For this review, take the finished solid that the model builds, in its own axes (mm). Coordinates: 2 decimals unless noted, no trailing zeros. Loops run counter-clockwise (first coordinate to the right, second up) from the corner with the lowest first, then second, coordinate; pieces in that order, holes last.
```python
from build123d import *

# Parameters (mm, degrees)
F1_DEPTH     = 2
F3_DEPTH     = 40
F4_T1_DEPTH  = 40
F4_T3_DEPTH  = 90
F4_T5_DEPTH  = 20
F4_T8_ANGLE  = 90
F4_T10_ANGLE = 90
F4_T12_ANGLE = 90
F4_T14_ANGLE = 90
F4_T15_DEPTH = 20
F4_T17_DEPTH = 34.8706177507
F4_T19_DEPTH = 34.8706177507
F4_T22_ANGLE = 90
F4_T24_ANGLE = 90
F4_T26_ANGLE = 90
F4_T28_ANGLE = 90
F4_T32_ANGLE = 67.9058899257
F4_S33_R     = 4
F4_T34_DEPTH = 6
F4_T38_ANGLE = 67.9058899257
F4_S39_R     = 4
F4_T40_DEPTH = 6
F4_T42_ANGLE = 2.1985680139
F4_T44_ANGLE = 2.1985680139
F4_T46_ANGLE = 145.4380511244
F4_T48_ANGLE = 145.4380511244
F5_W         = 47.7962438017
F5_H         = 14.3843935803
F6_DEPTH     = 25
F7_W         = 52.0751457661
F7_H         = 31.3179213554
F8_DEPTH     = 25


# Not quite as in the source:
# - a fillet or chamfer that OpenCascade refuses, or shapes differently, is made with other operations: its cross-section is extruded or revolved along the edge and cut away or added


with BuildPart() as f1:
    # F0 (on Top) → F1 (new body)
    with BuildSketch(Plane.XY):
        with BuildLine():
            Line((45, 20), (-45, 20))
            ThreePointArc((-45, 20), (-52.0710678119, 17.0710678119), (-55, 10))
            Line((-55, 10), (-55, -10))
            ThreePointArc((-55, -10), (-52.0710678119, -17.0710678119), (-45, -20))
            Line((-45, -20), (45, -20))
            ThreePointArc((45, -20), (52.0710678119, -17.0710678119), (55, -10))
            Line((55, -10), (55, 10))
            ThreePointArc((55, 10), (52.0710678119, 17.0710678119), (45, 20))
        make_face()
    extrude(amount=F1_DEPTH)

    # F2 (on face) → F3 (join, through all)
    with BuildSketch(Plane(origin=(0, 20, 0), x_dir=(-1, 0, 0), z_dir=(0, 1, 0))):
        with BuildLine():
            ThreePointArc((2.7771054409, 7.1347622527), (0, 3), (-2.7771054409, 7.1347622527))
            ThreePointArc((-2.7771054409, 7.1347622527), (-3.0758368725, 7.6594328143), (-3.674432988, 7.5806777712))
            ThreePointArc((-3.674432988, 7.5806777712), (-3.9185059144, 6.8033127653), (-3.9999931862, 5.9926169097))
            ThreePointArc((-3.9999931862, 5.9926169097), (-6.509106512, 3.1485501635), (-10.1236877963, 2))
            Line((-10.1236877963, 2), (10.1236877963, 2))
            ThreePointArc((10.1236877963, 2), (6.509106512, 3.1485501635), (3.9999931862, 5.9926169097))
            ThreePointArc((3.9999931862, 5.9926169097), (3.9185059144, 6.8033127653), (3.674432988, 7.5806777712))
            ThreePointArc((3.674432988, 7.5806777712), (3.0758368725, 7.6594328143), (2.7771054409, 7.1347622527))
        make_face()
    extrude(amount=-F3_DEPTH)

    # F4: fillet of radius 0.3 on 22 edges, made by hand

    # F4_s2 → F4_t1 (join)
    with BuildSketch(Plane.XZ.offset(-20)):
        with BuildLine():
            ThreePointArc((10.1293822493, 2), (10.1236267648, 2.0000552144), (10.1178733989, 2.0002208373))
            ThreePointArc((10.1178733989, 2.0002208373), (10.120780575, 2.0001098236), (10.1236877963, 2))
            Line((10.1236877963, 2), (10.1293822493, 2))
        make_face()
        with BuildLine():
            ThreePointArc((-10.1293822493, 2), (-10.1236267648, 2.0000552144), (-10.1178733989, 2.0002208373))
            ThreePointArc((-10.1178733989, 2.0002208373), (-10.120780575, 2.0001098236), (-10.1236877963, 2))
            Line((-10.1236877963, 2), (-10.1293822493, 2))
        make_face()
    extrude(amount=F4_T1_DEPTH)

    # F4_s4 → F4_t3 (cut)
    with BuildSketch(Plane.YZ.offset(-45)):
        with BuildLine():
            ThreePointArc((20, 0.3), (19.9121320344, 0.0878679656), (19.7, 0))
            Line((19.7, 0), (20, 0))
            Line((20, 0), (20, 0.3))
        make_face()
        with BuildLine():
            ThreePointArc((-19.7, 0), (-19.9121320344, 0.0878679656), (-20, 0.3))
            Line((-20, 0.3), (-20, 0))
            Line((-20, 0), (-19.7, 0))
        make_face()
    extrude(amount=F4_T3_DEPTH, mode=Mode.SUBTRACT)

    # F4_s6 → F4_t5 (cut)
    with BuildSketch(Plane.XZ.offset(-10)):
        with BuildLine():
            ThreePointArc((-54.7, 0), (-54.9121320344, 0.0878679656), (-55, 0.3))
            Line((-55, 0.3), (-55, 0))
            Line((-55, 0), (-54.7, 0))
        make_face()
        with BuildLine():
            ThreePointArc((54.7, 0), (54.9121320344, 0.0878679656), (55, 0.3))
            Line((55, 0.3), (55, 0))
            Line((55, 0), (54.7, 0))
        make_face()
    extrude(amount=F4_T5_DEPTH, mode=Mode.SUBTRACT)

    # F4_s7 → F4_t8 (revolve, cut)
    with BuildSketch(Plane.YZ.offset(-45)):
        with BuildLine():
            ThreePointArc((20, 0.3), (19.9121320344, 0.0878679656), (19.7, 0))
            Line((19.7, 0), (20, 0))
            Line((20, 0), (20, 0.3))
        make_face()
    revolve(axis=Axis((-45, 10, 0), (0, 0, 1)), revolution_arc=F4_T8_ANGLE, mode=Mode.SUBTRACT)

    # F4_s9 → F4_t10 (revolve, cut)
    with BuildSketch(Plane.XZ.offset(10)):
        with BuildLine():
            ThreePointArc((-54.7, 0), (-54.9121320344, 0.0878679656), (-55, 0.3))
            Line((-55, 0.3), (-55, 0))
            Line((-55, 0), (-54.7, 0))
        make_face()
    revolve(axis=Axis((-45, -10, 0), (0, 0, 1)), revolution_arc=F4_T10_ANGLE, mode=Mode.SUBTRACT)

    # F4_s11 → F4_t12 (revolve, cut)
    with BuildSketch(Plane.YZ.offset(45)):
        with BuildLine():
            ThreePointArc((-19.7, 0), (-19.9121320344, 0.0878679656), (-20, 0.3))
            Line((-20, 0.3), (-20, 0))
            Line((-20, 0), (-19.7, 0))
        make_face()
    revolve(axis=Axis((45, -10, 0), (0, 0, 1)), revolution_arc=F4_T12_ANGLE, mode=Mode.SUBTRACT)

    # F4_s13 → F4_t14 (revolve, cut)
    with BuildSketch(Plane.XZ.offset(-10)):
        with BuildLine():
            ThreePointArc((55, 0.3), (54.9121320344, 0.0878679656), (54.7, 0))
            Line((54.7, 0), (55, 0))
            Line((55, 0), (55, 0.3))
        make_face()
    revolve(axis=Axis((45, 10, 0), (0, 0, 1)), revolution_arc=F4_T14_ANGLE, mode=Mode.SUBTRACT)

    # F4_s16 → F4_t15 (cut)
    with BuildSketch(Plane.XZ.offset(-10)):
        with BuildLine():
            ThreePointArc((54.7, 2), (54.9121320344, 1.9121320344), (55, 1.7))
            Line((55, 1.7), (55, 2))
            Line((55, 2), (54.7, 2))
        make_face()
        with BuildLine():
            ThreePointArc((-54.7, 2), (-54.9121320344, 1.9121320344), (-55, 1.7))
            Line((-55, 1.7), (-55, 2))
            Line((-55, 2), (-54.7, 2))
        make_face()
    extrude(amount=F4_T15_DEPTH, mode=Mode.SUBTRACT)

    # F4_s18 → F4_t17 (cut)
    with BuildSketch(Plane.YZ.offset(10.1293822493)):
        with BuildLine():
            ThreePointArc((-19.7, 2), (-19.9121320344, 1.9121320344), (-20, 1.7))
            Line((-20, 1.7), (-20, 2))
            Line((-20, 2), (-19.7, 2))
        make_face()
        with BuildLine():
            ThreePointArc((20, 1.7), (19.9121320344, 1.9121320344), (19.7, 2))
            Line((19.7, 2), (20, 2))
            Line((20, 2), (20, 1.7))
        make_face()
    extrude(amount=F4_T17_DEPTH, mode=Mode.SUBTRACT)

    # F4_s20 → F4_t19 (cut)
    with BuildSketch(Plane.YZ.offset(-45)):
        with BuildLine():
            ThreePointArc((-19.7, 2), (-19.9121320344, 1.9121320344), (-20, 1.7))
            Line((-20, 1.7), (-20, 2))
            Line((-20, 2), (-19.7, 2))
        make_face()
        with BuildLine():
            ThreePointArc((20, 1.7), (19.9121320344, 1.9121320344), (19.7, 2))
            Line((19.7, 2), (20, 2))
            Line((20, 2), (20, 1.7))
        make_face()
    extrude(amount=F4_T19_DEPTH, mode=Mode.SUBTRACT)

    # F4_s21 → F4_t22 (revolve, cut)
    with BuildSketch(Plane.XZ.offset(-10)):
        with BuildLine():
            ThreePointArc((54.7, 2), (54.9121320344, 1.9121320344), (55, 1.7))
            Line((55, 1.7), (55, 2))
            Line((55, 2), (54.7, 2))
        make_face()
    revolve(axis=Axis((45, 10, 2), (0, 0, 1)), revolution_arc=F4_T22_ANGLE, mode=Mode.SUBTRACT)

    # F4_s23 → F4_t24 (revolve, cut)
    with BuildSketch(Plane.YZ.offset(45)):
        with BuildLine():
            ThreePointArc((-19.7, 2), (-19.9121320344, 1.9121320344), (-20, 1.7))
            Line((-20, 1.7), (-20, 2))
            Line((-20, 2), (-19.7, 2))
        make_face()
    revolve(axis=Axis((45, -10, 2), (0, 0, 1)), revolution_arc=F4_T24_ANGLE, mode=Mode.SUBTRACT)

    # F4_s25 → F4_t26 (revolve, cut)
    with BuildSketch(Plane.XZ.offset(10)):
        with BuildLine():
            ThreePointArc((-54.7, 2), (-54.9121320344, 1.9121320344), (-55, 1.7))
            Line((-55, 1.7), (-55, 2))
            Line((-55, 2), (-54.7, 2))
        make_face()
    revolve(axis=Axis((-45, -10, 2), (0, 0, 1)), revolution_arc=F4_T26_ANGLE, mode=Mode.SUBTRACT)

    # F4_s27 → F4_t28 (revolve, cut)
    with BuildSketch(Plane.YZ.offset(-45)):
        with BuildLine():
            ThreePointArc((20, 1.7), (19.9121320344, 1.9121320344), (19.7, 2))
            Line((19.7, 2), (20, 2))
            Line((20, 2), (20, 1.7))
        make_face()
    revolve(axis=Axis((-45, 10, 2), (0, 0, 1)), revolution_arc=F4_T28_ANGLE, mode=Mode.SUBTRACT)


with BuildPart() as f4_tool30:
    # F4_s31 → F4_t32 (revolve)
    with BuildSketch(Plane(origin=(-1.7091793366, 0, 4.7227038559), x_dir=(0, 1, 0), z_dir=(-0.3403063894, 0, 0.9403146076))):
        with BuildLine():
            ThreePointArc((20, -5.4610241004), (19.9121320344, -5.6731561348), (19.7, -5.7610241004))
            Line((19.7, -5.7610241004), (20, -5.7610241004))
            Line((20, -5.7610241004), (20, -5.4610241004))
        make_face()
    revolve(axis=Axis((10.3905055755, 20, 9.1016638887), (0, -1, 0)), revolution_arc=F4_T32_ANGLE)

    # F4_s33 → F4_t34 (cut, symmetric)
    with BuildSketch(Plane.XZ.offset(-19.7)):
        with Locations((0, 6)):
            Circle(F4_S33_R)
    extrude(amount=F4_T34_DEPTH, both=True, mode=Mode.SUBTRACT)


with BuildPart() as f1_1:
    add(f1.part)

    # F4_t29: cut F4_tool30
    add(f4_tool30.part, mode=Mode.SUBTRACT)


with BuildPart() as f4_tool36:
    # F4_s37 → F4_t38 (revolve)
    with BuildSketch(Plane(origin=(-10.0263051977, 0, -0.3849208379), x_dir=(0, 1, 0), z_dir=(-0.9992638755, 0, -0.0383628346))):
        with BuildLine():
            ThreePointArc((20, -2.0868987298), (19.9121320344, -2.2990307641), (19.7, -2.3868987298))
            Line((19.7, -2.3868987298), (20, -2.3868987298))
            Line((20, -2.3868987298), (20, -2.0868987298))
        make_face()
    revolve(axis=Axis((-10.3905055755, 20, 9.1016638887), (0, -1, 0)), revolution_arc=F4_T38_ANGLE)

    # F4_s39 → F4_t40 (cut, symmetric)
    with BuildSketch(Plane.XZ.offset(-19.7)):
        with Locations((0, 6)):
            Circle(F4_S39_R)
    extrude(amount=F4_T40_DEPTH, both=True, mode=Mode.SUBTRACT)


with BuildPart() as f1_2:
    add(f1_1.part)

    # F4_t35: cut F4_tool36
    add(f4_tool36.part, mode=Mode.SUBTRACT)

    # F4_s41 → F4_t42 (revolve, cut)
    with BuildSketch(Plane.YZ.offset(-10.1293822493)):
        with BuildLine():
            ThreePointArc((20, 1.7), (19.9121320344, 1.9121320344), (19.7, 2))
            Line((19.7, 2), (20, 2))
            Line((20, 2), (20, 1.7))
        make_face()
    revolve(axis=Axis((-10.1293822493, 20, 2.3), (0, -1, 0)), revolution_arc=F4_T42_ANGLE, mode=Mode.SUBTRACT)

    # F4_s43 → F4_t44 (revolve, cut)
    with BuildSketch(Plane.YZ.offset(10.1293822493)):
        with BuildLine():
            ThreePointArc((20, 1.7), (19.9121320344, 1.9121320344), (19.7, 2))
            Line((19.7, 2), (20, 2))
            Line((20, 2), (20, 1.7))
        make_face()
    revolve(axis=Axis((10.1293822493, 20, 2.3), (0, 1, 0)), revolution_arc=F4_T44_ANGLE, mode=Mode.SUBTRACT)

    # F4_s45 → F4_t46 (revolve, cut)
    with BuildSketch(Plane.YZ.offset(-10.1293822493)):
        with BuildLine():
            ThreePointArc((-19.7, 2), (-19.9121320344, 1.9121320344), (-20, 1.7))
            Line((-20, 1.7), (-20, 2))
            Line((-20, 2), (-19.7, 2))
        make_face()
    revolve(axis=Axis((-10.1293822493, -20, 2.3), (0, -1, 0)), revolution_arc=F4_T46_ANGLE, mode=Mode.SUBTRACT)

    # F4_s47 → F4_t48 (revolve, cut)
    with BuildSketch(Plane.YZ.offset(10.1293822493)):
        with BuildLine():
            ThreePointArc((-19.7, 2), (-19.9121320344, 1.9121320344), (-20, 1.7))
            Line((-20, 1.7), (-20, 2))
            Line((-20, 2), (-19.7, 2))
        make_face()
    revolve(axis=Axis((10.1293822493, -20, 2.3), (0, 1, 0)), revolution_arc=F4_T48_ANGLE, mode=Mode.SUBTRACT)

    # F5 (on face) → F6 (cut)
    with BuildSketch(Plane.XY.offset(2)):
        with Locations((-34.5203755423, 13.9260510914)):
            Rectangle(F5_W, F5_H)
        Polygon((-10.6222536415, 6.7338543013), (-58.4184974432, 6.7338543013), (-58.4184974432, -28.1346440315), (65.8517405391, -28.1346440315), (65.8517405391, 6.7338543013), (58.4184974432, 6.7338543013), (10.6222536415, 6.7338543013), align=None)
        with Locations((34.5203755423, 13.9260510914)):
            Rectangle(F5_W, F5_H)
    extrude(amount=-F6_DEPTH, mode=Mode.SUBTRACT)

    # F7 (on Top) → F8 (cut)
    with BuildSketch(Plane.XY):
        with Locations((-5.8881500736, -7.0132566616)):
            Rectangle(F7_W, F7_H)
    extrude(amount=F8_DEPTH, mode=Mode.SUBTRACT)


solid = f1_2.part
```
Q1. Wall thickness on probe 1 along X at (y, z) = (12.75, 6); probe 2 along Z at (x, y) = (0, 16.5); probe 3 along X at (y, z) = (19, 5.5): over which ranges is each line inside the solid? List them lowest first.
Q2. For pin 1 Ø3.5 at (x, z) = (0, 6) entering from +Y; pin 2 Ø1 at (x, y) = (2, 13) entering from +Z; pin 3 Ø2 at (y, z) = (10.5, 6) entering from -X; pin 4 Ø0.5 at (x, y) = (10.5, 16.5) entering from +Z, all flat-tipped, find the tip position at first contact; note any pin that passes through.
Q3. The part is to be moulded in two halves that separate along X. For faces 1 (the face through (-10.622, 14, 1)), 2 (the face through (10.622, 14, 1)), 3 (the face through (3.068, 14.402, 7.655)), say which applies: +X half, -X half, draft (parallel to the pull), parting line (faces both ways), or undercut.
Q4. Consider section A-A (z = 6.75). State the section outline as (x, y) points, then the cut area to 3 significant figures.
Q5. Consider section B-B (x = 0). State the section outline as (y, z) points, then the cut area to 3 significant figures.
Model answer:
1. probe 1: x = -4 to -3, 3 to 4
1. probe 2: z = 0 to 3
1. probe 3: x = -4.26 to -2.96, 2.96 to 4.26
2. pin 1: passes through
2. pin 2: stops at z = 4.34
2. pin 3: stops at x = -4.59
2. pin 4: stops at z = 2
3. face 1: -X half
3. face 2: +X half
3. face 3: undercut
4. outline: (-3.93, 8.65) - (-2.9, 8.65) - (-2.9, 20) - (-3.93, 20) - close; (2.9, 8.65) - (3.93, 8.65) - (3.93, 20) - (2.9, 20) - close
4. area: 23.3 mm2
5. outline: (8.65, 0) - (19.7, 0) arc R0.3 ccw to (20, 0.3) - (20, 3) - (8.65, 3) - close
5. area: 34.0 mm2
